Could you check a few things on this model? Use its own coordinates, in mm. Face numbers are marked on the shaded views. A direction names the side the tool comes from. Coordinates: 2 decimals unless noted, no trailing zeros. Order: outer loops, then holes, each group sorted by start corner. A loop starts at its lowest first (then second) coordinate and runs counter-clockwise, first axis right, second up. Notation, with made-up numbers: M -23.5,15 L 20.5,15 A13 cw 20.5,36 Z; hole C 47,-1.5 d8. An arc over 180 degrees is marked long. Put each result on its own line as item: value. Start each with the question number.
```python
from build123d import *

# Parameters (mm, degrees)
SKETCH_1_W          = 67
SKETCH_1_H          = 94
SKETCH_1_R          = 1.6
EXTRUDE_1_DEPTH     = 2
SKETCH_1_3_W        = 67
SKETCH_1_3_H        = 94
SKETCH_1_3_W_2      = 63
SKETCH_1_3_H_2      = 90
EXTRUDE_2_DEPTH     = 25
EXTRUDE_START       = 5
SKETCH_1_4_R        = 1.6
SKETCH_1_4_R_2      = 5
EXTRUDE_3_DEPTH     = 5
CUT_EXTRUDE_1_REACH = 115.248
SKETCH_2_W          = 55
SKETCH_2_H          = 19
FILLET_7_R          = 5
FILLET_8_R          = 1
FILLET_9_R          = 6
FILLET_11_R         = 6


with BuildPart() as part:
    # Эскиз1 → Бобышка-Вытянуть1 (new body)
    with BuildSketch(Plane(origin=(0, 0, 0), x_dir=(1, 0, 0), z_dir=(0, 1, 0))):
        with Locations((24.5, 39)):
            Rectangle(SKETCH_1_W, SKETCH_1_H)
        with Locations(Location((0, 0, 0), (0, 0, 270))):
            Circle(SKETCH_1_R, mode=Mode.SUBTRACT)
        with Locations(Location((49, 0, 0), (0, 0, 270))):
            Circle(SKETCH_1_R, mode=Mode.SUBTRACT)
        with Locations(Location((49, 58, 0), (0, 0, 270))):
            Circle(SKETCH_1_R, mode=Mode.SUBTRACT)
        with Locations(Location((0, 58, 0), (0, 0, 270))):
            Circle(SKETCH_1_R, mode=Mode.SUBTRACT)
        with Locations(Location((23, 58, 0), (0, 0, 270))):
            Circle(SKETCH_1_R, mode=Mode.SUBTRACT)
        with Locations(Location((23, 0, 0), (0, 0, 270))):
            Circle(SKETCH_1_R, mode=Mode.SUBTRACT)
    extrude(amount=-EXTRUDE_1_DEPTH)

    # Эскиз1<3> → Бобышка-Вытянуть2 (add)
    with BuildSketch(Plane(origin=(0, 0, 0), x_dir=(1, 0, 0), z_dir=(0, 1, 0))):
        with Locations((24.5, 39)):
            Rectangle(SKETCH_1_3_W, SKETCH_1_3_H)
        with Locations((24.5, 39)):
            Rectangle(SKETCH_1_3_W_2, SKETCH_1_3_H_2, mode=Mode.SUBTRACT)
    extrude(amount=EXTRUDE_2_DEPTH)

    # Эскиз1<4> → Бобышка-Вытянуть3 (add)
    # profile 1 of 6: a face of its own
    with BuildSketch(Plane(origin=(0, 0, 0), x_dir=(1, 0, 0), z_dir=(0, 1, 0)).offset(EXTRUDE_START)):
        with BuildLine():
            Line((-7, 5), (-7, -6))
            Line((-7, -6), (5, -6))
            Line((5, -6), (5, 0))
            ThreePointArc((5, 0), (3.535533906, 3.535533906), (0, 5))
            Line((0, 5), (-7, 5))
        make_face()
        with Locations(Location((0, 0, 0), (0, 0, 270))):
            Circle(SKETCH_1_4_R, mode=Mode.SUBTRACT)
    # profile 2 of 6: a face of its own
    with BuildSketch(Plane(origin=(0, 0, 0), x_dir=(1, 0, 0), z_dir=(0, 1, 0)).offset(EXTRUDE_START)):
        with BuildLine():
            Line((18, 0), (18, -6))
            Line((18, -6), (28, -6))
            Line((28, -6), (28, 0))
            ThreePointArc((28, 0), (23, 5), (18, 0))
        make_face()
        with Locations(Location((23, 0, 0), (0, 0, 270))):
            Circle(SKETCH_1_4_R, mode=Mode.SUBTRACT)
    # profile 3 of 6: a face of its own
    with BuildSketch(Plane(origin=(0, 0, 0), x_dir=(1, 0, 0), z_dir=(0, 1, 0)).offset(EXTRUDE_START)):
        with BuildLine():
            Line((-7, 63), (-7, 53))
            Line((-7, 53), (0, 53))
            ThreePointArc((0, 53), (5, 58), (0, 63))
            Line((0, 63), (-7, 63))
        make_face()
        with Locations(Location((0, 58, 0), (0, 0, 270))):
            Circle(SKETCH_1_4_R, mode=Mode.SUBTRACT)
    # profile 4 of 6: a face of its own
    with BuildSketch(Plane(origin=(0, 0, 0), x_dir=(1, 0, 0), z_dir=(0, 1, 0)).offset(EXTRUDE_START)):
        with BuildLine():
            Line((44, 0), (44, -6))
            Line((44, -6), (56, -6))
            Line((56, -6), (56, 5))
            Line((56, 5), (49, 5))
            ThreePointArc((49, 5), (45.464466094, 3.535533906), (44, 0))
        make_face()
        with Locations(Location((49, 0, 0), (0, 0, 270))):
            Circle(SKETCH_1_4_R, mode=Mode.SUBTRACT)
    # profile 5 of 6: a face of its own
    with BuildSketch(Plane(origin=(0, 0, 0), x_dir=(1, 0, 0), z_dir=(0, 1, 0)).offset(EXTRUDE_START)):
        with BuildLine():
            Line((56, 53), (56, 63))
            Line((56, 63), (49, 63))
            ThreePointArc((49, 63), (44, 58), (49, 53))
            Line((49, 53), (56, 53))
        make_face()
        with Locations(Location((49, 58, 0), (0, 0, 270))):
            Circle(SKETCH_1_4_R, mode=Mode.SUBTRACT)
    # profile 6 of 6: a face of its own
    with BuildSketch(Plane(origin=(0, 0, 0), x_dir=(1, 0, 0), z_dir=(0, 1, 0)).offset(EXTRUDE_START)):
        with Locations(Location((23, 58, 0), (0, 0, 270))):
            Circle(SKETCH_1_4_R_2)
        with Locations(Location((23, 58, 0), (0, 0, 270))):
            Circle(SKETCH_1_4_R, mode=Mode.SUBTRACT)
    extrude(amount=-EXTRUDE_3_DEPTH)

    # Эскиз2 → Вырез-Вытянуть1 (cut, up to next)
    with BuildSketch(Plane(origin=(0, 0, -86), x_dir=(-1, 0, 0), z_dir=(0, 0, -1)), mode=Mode.PRIVATE) as cut_extrude_1_sk1:
        with Locations((-24.5, 15.5)):
            Rectangle(SKETCH_2_W, SKETCH_2_H)
    cut_extrude_1_tool1 = extrude(cut_extrude_1_sk1.sketch, amount=-CUT_EXTRUDE_1_REACH, mode=Mode.PRIVATE) & part.part
    add(cut_extrude_1_tool1.solids().sort_by_distance((24.5, 15.5, -86))[0], mode=Mode.SUBTRACT)

    # Скругление7
    fillet_7_edges = [part.edges().sort_by_distance(p)[0] for p in [
        (56, 12.5, -84),
        (-7, 12.5, -84),
        (56, 15, 6),
        (-7, 15, 6),
    ]]
    fillet(fillet_7_edges, radius=FILLET_7_R)

    # Скругление8
    fillet_8_edges = [part.edges().sort_by_distance(p)[0] for p in [
        (5, 0, 3),
        (36, 0, 6),
        (23, 0, -5),
        (18, 0, 3),
        (28, 0, 3),
        (56, 0, -29),
        (45.464466094, 0, -3.535533906),
        (44, 0, 3),
        (52.5, 0, -5),
        (24.5, 0, -84),
        (-5.535533906, 0, -82.535533906),
        (54.535533906, 0, -82.535533906),
        (-7, 0, -71),
        (5, 0, -58),
        (-3.5, 0, -63),
        (-3.5, 0, -53),
        (23, 0, -63),
        (56, 0, -71),
        (44, 0, -58),
        (52.5, 0, -53),
        (52.5, 0, -63),
        (-7, 0, -29),
        (11.5, 0, 6),
        (3.535533906, 0, -3.535533906),
        (-3.5, 0, -5),
    ]]
    fillet(fillet_8_edges, radius=FILLET_8_R)

    # Скругление9
    fillet_9_edges = [part.edges().sort_by_distance(p)[0] for p in [
        (58, 11.5, 8),
        (-9, 11.5, 8),
        (-9, -2, -39),
        (24.5, -2, 8),
        (58, -2, -39),
        (24.5, -2, -86),
    ]]
    fillet(fillet_9_edges, radius=FILLET_9_R)

    # Скругление11
    # the kernel refuses this fillet: 6 mm, written as the material it takes off along each edge
    with BuildSketch(Plane(origin=(-3, 4, -80), x_dir=(-1, 0, 0), z_dir=(0, 0, -1))) as fillet_11_piece_1_section:
        Polygon((0, 0), (FILLET_11_R, 0), (FILLET_11_R, -FILLET_11_R), (0, -FILLET_11_R), align=None)
    fillet_11_piece_1 = extrude(amount=FILLET_11_R, mode=Mode.PRIVATE)
    fillet_11_piece_1 = fillet_11_piece_1 - Plane(origin=(-3, 4, -80), x_dir=(0.7071067811865475, 0.7071067811865475, 0), z_dir=(0, 0, -1)) * Sphere(FILLET_11_R, mode=Mode.PRIVATE)
    add(fillet_11_piece_1, mode=Mode.SUBTRACT)
    with BuildSketch(Plane(origin=(52, 4, -80), x_dir=(0, 0, -1), z_dir=(1, 0, 0))) as fillet_11_piece_2_section:
        Polygon((0, 0), (FILLET_11_R, 0), (FILLET_11_R, -FILLET_11_R), (0, -FILLET_11_R), align=None)
    fillet_11_piece_2 = extrude(amount=FILLET_11_R, mode=Mode.PRIVATE)
    fillet_11_piece_2 = fillet_11_piece_2 - Plane(origin=(52, 4, -80), x_dir=(0, 0.7071067811865475, 0.7071067811865475), z_dir=(1, 0, 0)) * Sphere(FILLET_11_R, mode=Mode.PRIVATE)
    add(fillet_11_piece_2, mode=Mode.SUBTRACT)
    with BuildSketch(Plane(origin=(-9, 40, -86), x_dir=(1, 0, 0), z_dir=(0, -1, 0)), Plane(origin=(58, 40, -86), x_dir=(0, 0, 1), z_dir=(0, -1, 0))) as fillet_11_piece_3:
        with BuildLine():
            CenterArc((FILLET_11_R, FILLET_11_R), FILLET_11_R, 180, 90)
            Line((0, FILLET_11_R), (0, 0))
            Line((0, 0), (FILLET_11_R, 0))
        make_face()
    extrude(amount=36, mode=Mode.SUBTRACT)


solid = part.part
```
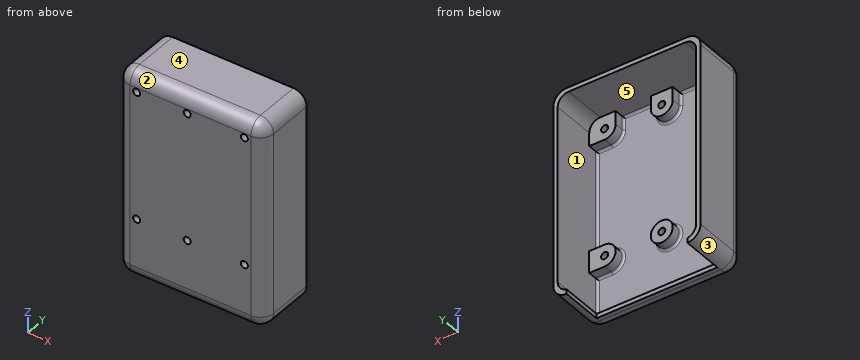
Item 1: For the marked faces 4 and 5, which set-ups out of +Z, -Z, +X, -X, +Y, -Y let a thin tool reach every point of the face, with its end or its side?
Item 2: For pin 1 Ø4.5 at (x, y) = (-5, 4) entering from -Z; pin 2 Ø3 at (x, z) = (0, -58) entering from +Y; pin 3 Ø5 at (x, z) = (11.5, -40) entering from +Y; pin 4 Ø1.2 at (x, y) = (52.5, 3) entering from +Z, each with a flat end and sliding along its axis, tell me the tip position at first contact or that it passes through.
Item 3: If we section it at A-A on x = 23: Write out the boundary of the cut face in (y, z).
Item 4: I need wall thicknesses on probe 1 along X at (y, z) = (3.75, 0); probe 2 along X at (y, z) = (20, -7); probe 3 along X at (y, z) = (1.5, 0). Which ranges of each line are inside material? Lowest first, please.
Item 5: If we section it at B-B on z = -58: State how many separate pieces and enclosed holes the cut face has, then the cut area to 3 significant figures.
Item 6: If we section it at C-C on y = 9.5: Write out the boundary of the cut face in (x, z), then the cut area to 3 significant figures.
Item 7: If we mould it in two halves opening along Z, with no side actions, what happens to the marked faces 1, 2 and 3? For each: released by +Z, released by -Z, zero draft, split by the parting line, or undercut.
Item 8: If we section it at D-D on z = -44.5: Write out the boundary of the cut face in (x, y), then the cut area to 3 significant figures.
Geometry check:
1. face 4: +Z, +X, -X, +Y, -Y
1. face 5: +Y
2. pin 1: stops at z = -86
2. pin 2: passes through
2. pin 3: stops at y = 0
2. pin 4: stops at z = 7.98
3. outline: M -2,-80 A6 ccw 4,-86 L 6,-86 L 6,-84 L 1,-84 A1 cw 0,-83 L 0,-64 A1 cw 1,-63 L 5,-63 L 5,-59.6 L -2,-59.6 Z; M -2,-56.4 L 5,-56.4 L 5,-53 L 1,-53 A1 cw 0,-52 L 0,-6 A1 cw 1,-5 L 5,-5 L 5,-1.6 L -2,-1.6 Z; M -2,1.6 L 5,1.6 L 5,6 L 25,6 L 25,8 L 4,8 A6 ccw -2,2 Z
4. probe 1: x = -8.99 to -1.6, 1.6 to 5, 18 to 21.4, 24.6 to 28, 44 to 47.4, 50.6 to 57.99
4. probe 2: x = -9 to -7, 56 to 58
4. probe 3: x = -8.45 to -1.6, 1.6 to 5, 18 to 21.4, 24.6 to 28, 44 to 47.4, 50.6 to 57.45
5. separate pieces: 4
5. enclosed holes: 0
5. area: 322 mm²
6. outline: M -9,-80 A6 ccw -3,-86 L -3,-83.9 A5 cw -7,-79 L -7,1 A5 cw -2,6 L 51,6 A5 cw 56,1 L 56,-79 A5 cw 52,-83.9 L 52,-86 A6 ccw 58,-80 L 58,2 A6 ccw 52,8 L -3,8 A6 ccw -9,2 Z
6. area: 508 mm²
7. face 1: undercut
7. face 2: released by +Z
7. face 3: released by -Z
8. outline: M -9,4 A6 ccw -3,-2 L 52,-2 A6 ccw 58,4 L 58,25 L 56,25 L 56,1 A1 cw 55,0 L -6,0 A1 cw -7,1 L -7,25 L -9,25 Z
8. area: 219 mm²
